Could you check a few things on this model? Use its own coordinates, in mm. Face numbers are marked on the shaded views. A direction names the side the tool comes from. Round coordinates to 2 decimals unless told otherwise and drop trailing zeros. Loops run counter-clockwise (first coordinate to the right, second up) from the corner with the lowest first, then second, coordinate; pieces in that order, holes last. Notation, with made-up numbers: (88.5, 72) -> (110.5, 72) arc R18 ccw to (110.5, 95) -> close; hole circle Ø8 at (-21.75, -7.5). An arc over 180 degrees is marked (long way). One line per item, written item: value.
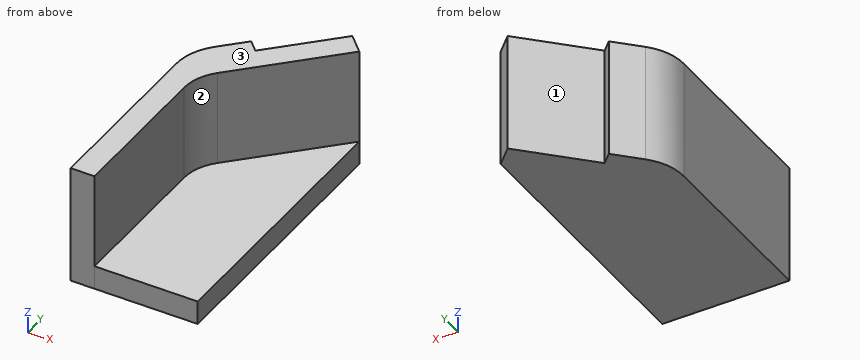
from build123d import *

# Parameters (mm, degrees)
BOSS_EXTRUDE1_DEPTH = 5
BOSS_EXTRUDE2_START = -2
BOSS_EXTRUDE2_DEPTH = 2


with BuildPart() as part:
    # Sketch2 → Boss-Extrude1 (new, symmetric)
    with BuildSketch(Plane(origin=(-44.395698949, 24.726348819, -28.895), x_dir=(0.707106781186551, -0.7071067811865441, 0), z_dir=(0, 0, 1))):
        with BuildLine():
            Line((5.05, 7), (7.05, 7))
            Line((7.05, 7), (7.05, -3.589034995))
            ThreePointArc((7.05, -3.589034995), (7.35448187, -5.119768725), (8.221572875, -6.41746212))
            Line((8.221572875, -6.41746212), (17.247782384, -15.443671629))
            Line((17.247782384, -15.443671629), (15.833568821, -16.857885191))
            Line((15.833568821, -16.857885191), (5.175341815, -6.199658185))
            ThreePointArc((5.175341815, -6.199658185), (4.194445115, -4.731642531), (3.85, -3))
            Line((3.85, -3), (3.85, -0.25))
            Line((3.85, -0.25), (5.05, -0.25))
            Line((5.05, -0.25), (5.05, 7))
        make_face()
    extrude(amount=BOSS_EXTRUDE1_DEPTH, both=True)

    # Sketch3 → Boss-Extrude2 (add)
    with BuildSketch(Plane(origin=(0, 0, -33.895), x_dir=(-1, 0, 0), z_dir=(0, 0, -1)).offset(BOSS_EXTRUDE2_START)):
        with BuildLine():
            Line((34.460848673, 24.69099348), (34.460848673, 1.61))
            Line((34.460848673, 1.61), (43.12, 1.61))
            Line((43.12, 1.61), (43.12, 14.374987904))
            ThreePointArc((43.12, 14.374987904), (42.81551813, 15.905721633), (41.948427125, 17.203415028))
            Line((41.948427125, 17.203415028), (34.460848673, 24.69099348))
        make_face()
    extrude(amount=BOSS_EXTRUDE2_DEPTH)


solid = part.part
(1) If we section it at D-D, the plane z = -33: Please give me the cut outline in (x, y) (3 decimals), then the cut area to 3 significant figures.
Recorded:
outline: (-45.12, 1.61) -> (-34.461, 1.61) -> (-34.461, 24.691) -> (-35.875, 26.105) -> (-41.002, 20.979) -> (-41.85, 21.827) -> (-43.795, 19.883) arc R4.525 ccw to (-45.12, 16.683) -> close
area: 223 mm²
(2) If we section it at C-C, the plane y = 5.5: Please give me the cut outline in (x, z) (3 decimals), then the cut area to 3 significant figures.
Recorded:
outline: (-45.12, -33.895) -> (-34.461, -33.895) -> (-34.461, -31.895) -> (-43.12, -31.895) -> (-43.12, -23.895) -> (-45.12, -23.895) -> close
area: 37.3 mm²
(3) If we section it at B-B, the plane z = -30.5: Please give me the cut outline in (x, y) (3 decimals).
Recorded:
outline: (-45.12, 1.61) -> (-43.12, 1.61) -> (-43.12, 14.375) arc R4 cw to (-41.948, 17.203) -> (-34.461, 24.691) -> (-35.875, 26.105) -> (-41.002, 20.979) -> (-41.85, 21.827) -> (-43.795, 19.883) arc R4.525 ccw to (-45.12, 16.683) -> close
(4) I'm going to push flat-ended pins straight in: pin 1 Ø3 at (y, z) = (16.5, -29.5) entering from +X; pin 2 Ø5 at (x, z) = (-41, -28) entering from +Y; pin 3 Ø2.5 at (x, y) = (-38, 8.5) entering from +Z (3 decimals). Where does each tip first touch, or does it pass through?
Recorded:
pin 1: x = -41.15
pin 2: y = 23.48
pin 3: z = -31.895
(5) If I drill on L1, parallel to Z at x = -42.5, y = 14.75 (3 decimals); L2, parallel to X at y = 4, z = -31.5; L3, parallel to Y at x = -35.75, z = -32, over which ranges is the centre line in solid material (lowest first)?
Recorded:
L1: -33.895 to -31.895
L2: -45.12 to -43.12
L3: 1.61 to 25.98
(6) If we section it at A-A, the plane y = 21.5: Please give me the cut outline in (x, z) (3 decimals).
Recorded:
outline: (-42.177, -33.895) -> (-41.523, -33.895) -> (-41.523, -23.895) -> (-42.177, -23.895) -> close; (-40.48, -33.895) -> (-34.461, -33.895) -> (-34.461, -31.895) -> (-37.652, -31.895) -> (-37.652, -23.895) -> (-40.48, -23.895) -> close
(7) For the marked faces 1, 2 and 3, which set-ups out of +Z, -Z, +X, -X, +Y, -Y let a thin tool reach every point of the face, with its end or its side?
Recorded:
face 1: +Z, -Z, +Y
face 2: +Z, +X, -Y
face 3: +Z, +X, -X, +Y, -Y
